from build123d import *

# Parameters (mm, degrees)
SKETCH1_W               = 30.6846
SKETCH1_H               = 15
BOSS_EXTRUDE1_DEPTH     = 3
SKETCH2_W               = 3
SKETCH2_H               = 15
BOSS_EXTRUDE2_DEPTH     = 17
SKETCH4_W               = 3.175
SKETCH4_H               = 3
BOSS_EXTRUDE3_DEPTH     = 15
CUT_EXTRUDE1_DEPTH      = 43.601409744
CUT_EXTRUDE1_DEPTH_BACK = 43.601409744
SKETCH3_R               = 2.358188849
SKETCH5_W               = 5
SKETCH5_H               = 20
BOSS_EXTRUDE4_DEPTH     = 3


with BuildPart() as part:
    # Sketch1 → Boss-Extrude1 (new body)
    with BuildSketch(Plane(origin=(0, 0, 0), x_dir=(1, 0, 0), z_dir=(0, 1, 0))):
        Rectangle(SKETCH1_W, SKETCH1_H)
    extrude(amount=BOSS_EXTRUDE1_DEPTH)

    # Sketch2 → Boss-Extrude2 (add)
    with BuildSketch(Plane(origin=(0, 3, 0), x_dir=(1, 0, 0), z_dir=(0, 1, 0))):
        with Locations((-13.8423, 0)):
            Rectangle(SKETCH2_W, SKETCH2_H)
        with Locations((13.8423, 0)):
            Rectangle(SKETCH2_W, SKETCH2_H)
    extrude(amount=BOSS_EXTRUDE2_DEPTH)

    # Sketch4 → Boss-Extrude3 (add)
    with BuildSketch(Plane.XY.offset(7.5)):
        Polygon((-18.5173, 0), (-18.5173, 3), (-18.5173, 20), (-21.5173, 20), (-21.5173, 0), align=None)
        with Locations((-16.9298, 1.5)):
            Rectangle(SKETCH4_W, SKETCH4_H)
        with Locations((16.9298, 1.5)):
            Rectangle(SKETCH4_W, SKETCH4_H)
        Polygon((18.5173, 20), (18.5173, 3), (18.5173, 0), (21.5173, 0), (21.5173, 20), align=None)
    extrude(amount=-BOSS_EXTRUDE3_DEPTH)

    # Sketch3 → Cut-Extrude1 (cut, two sides: drawn at the far end of the back side and taken through both)
    with BuildSketch(Plane.ZY.offset(15.3423).offset(-CUT_EXTRUDE1_DEPTH_BACK)):
        with Locations((0, 11.477245264)):
            Circle(SKETCH3_R)
    extrude(amount=CUT_EXTRUDE1_DEPTH + CUT_EXTRUDE1_DEPTH_BACK, mode=Mode.SUBTRACT)

    # Sketch5 → Boss-Extrude4 (add)
    # profile 1 of 2: a face of its own
    with BuildSketch(Plane(origin=(0, 0, 0), x_dir=(-1, 0, 0), z_dir=(0, -1, 0))):
        with Locations((24.0173, -2.5)):
            Rectangle(SKETCH5_W, SKETCH5_H)
        with BuildLine():
            Line((25.6923, 4.5), (25.6923, -9.5))
            ThreePointArc((25.6923, -9.5), (24.0173, -11.175), (22.3423, -9.5))
            Line((22.3423, -9.5), (22.3423, 4.5))
            ThreePointArc((22.3423, 4.5), (24.0173, 6.175), (25.6923, 4.5))
        make_face(mode=Mode.SUBTRACT)
    # profile 2 of 2: a face of its own
    with BuildSketch(Plane(origin=(0, 0, 0), x_dir=(-1, 0, 0), z_dir=(0, -1, 0))):
        with Locations((-24.0173, -2.5)):
            Rectangle(SKETCH5_W, SKETCH5_H)
        with BuildLine():
            Line((-22.3423, 4.5), (-22.3423, -9.5))
            ThreePointArc((-22.3423, -9.5), (-24.0173, -11.175), (-25.6923, -9.5))
            Line((-25.6923, -9.5), (-25.6923, 4.5))
            ThreePointArc((-25.6923, 4.5), (-24.0173, 6.175), (-22.3423, 4.5))
        make_face(mode=Mode.SUBTRACT)
    extrude(amount=-BOSS_EXTRUDE4_DEPTH)


solid = part.part
Model file for the job. Use its own axes, mm. A direction names the side the tool comes from. Give positions to 0.01 mm unless a question says otherwise; leave off trailing zeros. Loops run counter-clockwise (first coordinate to the right, second up) from the corner with the lowest first, then second, coordinate; pieces in that order, holes last.
Item 1: Slice it at C-C (z = 8). Write the cut outline in (x, y), plus the area to 3 significant figures.
Check values:
outline: (-26.52, 0) - (-25.69, 0) - (-25.69, 3) - (-26.52, 3) - close; (-22.34, 0) - (-21.52, 0) - (-21.52, 3) - (-22.34, 3) - close; (21.52, 0) - (22.34, 0) - (22.34, 3) - (21.52, 3) - close; (25.69, 0) - (26.52, 0) - (26.52, 3) - (25.69, 3) - close
area: 9.90 mm2
Item 2: Slice it at D-D (y = 12.25). Give the number of separate pieces and of enclosed holes in the cut face, plus the area to 3 significant figures.
Check values:
separate pieces: 8
enclosed holes: 0
area: 127 mm2
Item 3: Drill centre lines: line 1 along X through (y, z) = (18.25, -2); line 2 along X through (y, z) = (2.75, 9.5); line 3 along X through (y, z) = (1.5, -0.5). Where is each one in solid material? Low to high.
Check values:
line 1: x = -21.52 to -18.52, -15.34 to -12.34, 12.34 to 15.34, 18.52 to 21.52
line 2: x = -26.52 to -25.69, -22.34 to -21.52, 21.52 to 22.34, 25.69 to 26.52
line 3: x = -26.52 to -25.69, -22.34 to 22.34, 25.69 to 26.52
Item 4: Which spindle directions (+Z, -Z, +X, -X, +Y, -Y) get a long thin tool onto all of the face, cutting with end or side? Do faces 4 (the face through (-1.8, 2.5, -7.5)), 5 (the face through (26, 3, 2)), 6 (the face through (20.038, 9.175, -0.511)), 7 (the face through (12.342, 9, 2)), 8 (the face through (23.98, 1.479, 11.175)). Say none if no direction does.
Check values:
face 4: -Z, +X, -X, +Y, -Y
face 5: +Z, -Z, +X, +Y
face 6: +X, -X
face 7: +Z, -Z, +Y
face 8: +Y, -Y
Item 5: Mould opens along Z. For faces 1 (the face through (-21.517, 14, 2)), 2 (the face through (0, 1, 7.5)), 3 (the face through (-19.996, 9.175, -0.511)) say: +Z half, -Z half, draft (parallel to the pull), parting line (faces both ways), or undercut.
Check values:
face 1: draft
face 2: +Z half
face 3: undercut
Item 6: Drop flat-ended pins along their axis: P1, Ø12, axis at x = -5, z = -1, coming from the +Y side; P2, Ø6, axis at y = 11.48, z = 0, coming from the -X side; P3, Ø6, axis at x = -10, y = 3.5, coming from the +Z side. Give the stop position or say it passes through.
Check values:
P1: stops at y = 3
P2: stops at x = -21.52
P3: stops at z = 7.5
Item 7: Slice it at B-B (z = 4.5). Write the cut outline in (x, y).
Check values:
outline: (-26.52, 0) - (-25.69, 0) - (-25.69, 3) - (-26.52, 3) - close; (-22.34, 0) - (22.34, 0) - (22.34, 3) - (21.52, 3) - (21.52, 20) - (18.52, 20) - (18.52, 3) - (15.34, 3) - (15.34, 20) - (12.34, 20) - (12.34, 3) - (-12.34, 3) - (-12.34, 20) - (-15.34, 20) - (-15.34, 3) - (-18.52, 3) - (-18.52, 20) - (-21.52, 20) - (-21.52, 3) - (-22.34, 3) - close; (25.69, 0) - (26.52, 0) - (26.52, 3) - (25.69, 3) - close
Item 8: Slice it at A-A (y = 1.5). Write the cut outline in (x, z) (3 decimals).
Check values:
outline: (-26.517, -7.5) - (26.517, -7.5) - (26.517, 12.5) - (21.517, 12.5) - (21.517, 7.5) - (-21.517, 7.5) - (-21.517, 12.5) - (-26.517, 12.5) - close; hole (-25.692, -4.5) arc R1.675 ccw to (-22.342, -4.5) - (-22.342, 9.5) arc R1.675 ccw to (-25.692, 9.5) - close; hole (22.342, -4.5) arc R1.675 ccw to (25.692, -4.5) - (25.692, 9.5) arc R1.675 ccw to (22.342, 9.5) - close
